Autodesk Fusion 360 part; units mm, degrees
sketch "Sketch1" plane through (0, 0, 0) normal (0, 0, 1) x (1, 0, 0)
  line L0 (0, 0) -> (40, 0)
  line L1 (40, 0) -> (40, 30)
  line L2 (40, 30) -> (0, 30)
  line L3 (0, 30) -> (0, 0)
  dimension "d1" = 40
  dimension "d2" = 30
extrude "Extrude1" add sketch "Sketch1" along normal blind 2
sketch "Sketch2" plane through (0, 0, 2) normal (0, 0, 1) x (-1, 0, 0)
  line L0 (0, -30) -> (0, 0)
  line L1 (0, 0) -> (-40, 0)
  line L2 (-40, 0) -> (-40, -30)
  line L3 (-40, -30) -> (0, -30)
  line L4 (-9, -30) -> (-10, -30)
  line L5 (-10, -30) -> (-10, 0)
  line L6 (-10, 0) -> (-9, 0)
  line L7 (-9, 0) -> (-9, -30)
  dimension "d5" = 1
  dimension "d6" = 30
  dimension "d7" = 9
extrude "Extrude2" cut sketch "Sketch2" against normal blind 1 contours L1 L3 L4 L5 L6 L7
sketch "Sketch4" plane through (0, 0, 0) normal (0, 0, -1) x (1, 0, 0)
  line L0 (0, 0) -> (0, -30)
  line L1 (0, -30) -> (40, -30)
  line L2 (40, -30) -> (40, 0)
  line L3 (40, 0) -> (0, 0)
  line L4 (40, 0) -> (38, 0)
  line L5 (38, 0) -> (38, -30)
  line L6 (38, -30) -> (40, -30)
  line L7 (40, -30) -> (40, 0)
extrude "Extrude3" add sketch "Sketch4" along normal blind 58 contours L1 L2 L3 L4 L5 L6 L7
extrude "Extrude4" add 1 faces at (0, 20, 0.6667) along direction (-1, 0, 0) blind 60
extrude "Extrude5" add 1 faces at (9.3333, 20, 1) along direction (0, 0, 1) blind 1
sketch "Sketch5" plane through (0, 0, 2) normal (0, 0, 1) x (-1, 0, 0)
  line L0 (-40, -30) -> (60, -30)
  line L1 (60, -30) -> (60, 0)
  line L2 (60, 0) -> (-40, 0)
  line L3 (-40, 0) -> (-40, -30)
  line L4 (11, 0) -> (10, 0)
  line L5 (10, 0) -> (10, -30)
  line L6 (10, -30) -> (11, -30)
  line L7 (11, -30) -> (11, 0)
  dimension "d18" = 1
  dimension "d19" = 30
  dimension "d20" = 49
extrude "Extrude6" cut sketch "Sketch5" along normal blind 1 contours L0 L2 L4 L5 L6 L7
sketch "Sketch6" plane through (0, 0, 2) normal (0, 0, 1) x (-1, 0, 0)
  line L0 (60, 0) -> (-40, 0)
  line L1 (-40, 0) -> (-40, -30)
  line L2 (-40, -30) -> (60, -30)
  line L3 (60, -30) -> (60, 0)
equation "d21 = mm"
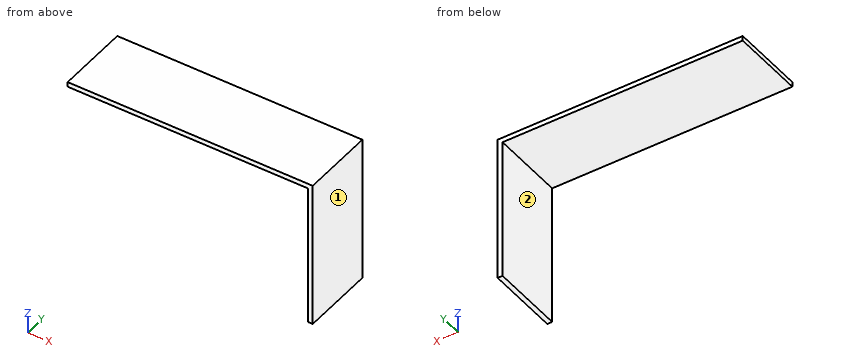
Model file for the job. Use its own axes, mm. Face numbers are marked on the shaded views. A direction names the side the tool comes from. Coordinates: 2 decimals unless noted, no trailing zeros. Write each loop counter-clockwise with the first axis right and the second up, starting at its lowest first coordinate (ties: lowest second). Pieces come first, ordered by that corner, then holes. Notation, with made-up numbers: (-27, -25.5) - (18, -25.5) arc R28 cw to (18, 8.5) - close; hole circle Ø7 at (40.25, 7). An arc over 180 degrees is marked (long way). One line per item, written item: value. Start each with the question number.
1. Slice it at C-C (x = 5). Write the cut outline in (y, z), plus the area to 3 significant figures.
2. Probe line 1 (Z direction, x = 0, y = 19.5); line 2 (X direction, y = 19.75, z = -31). List the from-to ranges inside material, lowest first. Write a range as from..to.
3. Flat gauge pins, fed straight in: pin 1 (8 mm diameter, centred on y = 17, z = -29.5, fed in from -X); pin 2 (3 mm diameter, centred on x = -43, y = 4, fed in from -Z). Where does each tip first touch, or does it go through?
4. Slice it at B-B (z = -52). Write the cut outline in (x, y), plus the area to 3 significant figures.
5. Slice it at A-A (y = 20.5). Write the cut outline in (x, z).
6. Tool access for the marked faces 1 and 2: list every direction of +Z, -Z, +X, -X, +Y, -Y with a clear straight run to the whole face (end or side of a thin tool).
Answers below:
1. outline: (0, 0) - (30, 0) - (30, 2) - (0, 2) - close
1. area: 60.0 mm^2
2. line 1: z = 0..2
2. line 2: x = 38..40
3. pin 1: stops at x = 38
3. pin 2: stops at z = 0
4. outline: (38, 0) - (40, 0) - (40, 30) - (38, 30) - close
4. area: 60.0 mm^2
5. outline: (-60, 0) - (38, 0) - (38, -58) - (40, -58) - (40, 2) - (-60, 2) - close
6. face 1: +Z, -Z, +X, +Y, -Y
6. face 2: -Z, -X, +Y, -Y
